```python
from build123d import *

# Parameters (mm, degrees)
OBJ1_R                     = 2.75
OBJ1_DEPTH                 = 8
OBJ2                     = 2.75
OBJ3                 = 8
OBJ4_PLACEMENT_ANGLE        = 90
TBOLT_SHAFT_R                    = 2
TBOLT_SHAFT_DEPTH                = 20
TBOLT_SHAFT_ROLL_ANGLE           = 90
UP_SEP_W                         = 16
UP_SEP_H                         = 1.2
UP_SEP_DEPTH                     = 13.8
SHAFT_HOLE_R                     = 4
SHAFT_HOLE_DEPTH                 = 16
SHAFT_HOLE_PITCH_ANGLE           = 90
TBOLT_HEAD_R                     = 3.85
TBOLT_HEAD_DEPTH                 = 5.4
TBOLT_HEAD_ROLL_ANGLE            = 90
SIDE_BOX_L_W                     = 14
SIDE_BOX_L_H                     = 12
SIDE_BOX_L_DEPTH                 = 26.8
SIDE_BOX_R_W                     = 14
SIDE_BOX_R_H                     = 12
SIDE_BOX_R_DEPTH                 = 26.8
TOTAL_BOX_W                      = 14
TOTAL_BOX_H                      = 42
TOTAL_BOX_DEPTH                  = 32.8
SK_SHAPE_W_HOLES_PLACEMENT_ANGLE = 90


with BuildPart() as obj1:
    # obj1 → obj1 (new body)
    with BuildSketch(Plane(origin=(7, -16, -1), x_dir=(1, 0, 0), z_dir=(0, 0, 1))):
        Circle(OBJ1_R)
    extrude(amount=OBJ1_DEPTH)


with BuildPart() as obj4:
    with BuildSketch(Plane(origin=(7, 16, -1), x_dir=(1, 0, 0), z_dir=(0, 0, 1))):
        Circle(OBJ2)
    extrude(amount=OBJ3)

    # obj4: union obj1
    add(obj1.part)


with BuildPart() as obj4_1:
    # obj4 placement: moved
    add(obj4.part.moved(Location((0, -7, 0))).rotate(Axis((0, -7, 0), (0, 0, 1)), OBJ4_PLACEMENT_ANGLE))


with BuildPart() as tbolt_shaft:
    # tbolt_shaft → tbolt_shaft (new body)
    with BuildSketch(Plane.XY):
        Circle(TBOLT_SHAFT_R)
    extrude(amount=TBOLT_SHAFT_DEPTH)


with BuildPart() as tbolt_shaft_1:
    # tbolt_shaft roll: moved
    add(tbolt_shaft.part.rotate(Axis((0, 0, 0), (1, 0, 0)), TBOLT_SHAFT_ROLL_ANGLE))


with BuildPart() as tbolt_shaft_2:
    # tbolt_shaft placement: moved
    add(tbolt_shaft_1.part.moved(Location((7, 10, 27.5))))


with BuildPart() as up_sep:
    # up_sep → up_sep (new body)
    with BuildSketch(Plane(origin=(-1, -0.6, 21), x_dir=(1, 0, 0), z_dir=(0, 0, 1))):
        with Locations((8, 0.6)):
            Rectangle(UP_SEP_W, UP_SEP_H)
    extrude(amount=UP_SEP_DEPTH)


with BuildPart() as shaft_hole:
    # shaft_hole → shaft_hole (new body)
    with BuildSketch(Plane.XY):
        Circle(SHAFT_HOLE_R)
    extrude(amount=SHAFT_HOLE_DEPTH)


with BuildPart() as shaft_hole_1:
    # shaft_hole pitch: moved
    add(shaft_hole.part.rotate(Axis((0, 0, 0), (0, 1, 0)), SHAFT_HOLE_PITCH_ANGLE))


with BuildPart() as shaft_hole_2:
    # shaft_hole placement: moved
    add(shaft_hole_1.part.moved(Location((-1, 0, 20))))


with BuildPart() as fuse_shaft_holes:
    # tbolt_head → tbolt_head (new body)
    with BuildSketch(Plane.XY):
        Circle(TBOLT_HEAD_R)
    extrude(amount=TBOLT_HEAD_DEPTH)


with BuildPart() as fuse_shaft_holes_1:
    # tbolt_head roll: moved
    add(fuse_shaft_holes.part.rotate(Axis((0, 0, 0), (1, 0, 0)), TBOLT_HEAD_ROLL_ANGLE))


with BuildPart() as fuse_shaft_holes_2:
    # tbolt_head placement: moved
    add(fuse_shaft_holes_1.part.moved(Location((7, 10, 27.5))))

    # fuse_shaft_holes: union tbolt_shaft, up_sep, shaft_hole
    add(tbolt_shaft_2.part)
    add(up_sep.part)
    add(shaft_hole_2.part)


with BuildPart() as side_box_l:
    # side_box_l → side_box_l (new body)
    with BuildSketch(Plane(origin=(0, -21, 6), x_dir=(1, 0, 0), z_dir=(0, 0, 1))):
        with Locations((7, 6)):
            Rectangle(SIDE_BOX_L_W, SIDE_BOX_L_H)
    extrude(amount=SIDE_BOX_L_DEPTH)


with BuildPart() as side_boxes:
    # side_box_r → side_box_r (new body)
    with BuildSketch(Plane(origin=(0, 9, 6), x_dir=(1, 0, 0), z_dir=(0, 0, 1))):
        with Locations((7, 6)):
            Rectangle(SIDE_BOX_R_W, SIDE_BOX_R_H)
    extrude(amount=SIDE_BOX_R_DEPTH)

    # side_boxes: union side_box_l
    add(side_box_l.part)


with BuildPart() as sky_x_y0:
    # total_box → total_box (new body)
    with BuildSketch(Plane(origin=(0, -21, 0), x_dir=(1, 0, 0), z_dir=(0, 0, 1))):
        with Locations((7, 21)):
            Rectangle(TOTAL_BOX_W, TOTAL_BOX_H)
    extrude(amount=TOTAL_BOX_DEPTH)

    # sk_shape: cut side_boxes
    add(side_boxes.part, mode=Mode.SUBTRACT)

    # sk_shape_w_holes: cut fuse_shaft_holes
    add(fuse_shaft_holes_2.part, mode=Mode.SUBTRACT)


with BuildPart() as sky_x_y0_1:
    # sk_shape_w_holes placement: moved
    add(sky_x_y0.part.moved(Location((0, -7, 0))).rotate(Axis((0, -7, 0), (0, 0, 1)), SK_SHAPE_W_HOLES_PLACEMENT_ANGLE))

    # sky_x_y0: cut obj4
    add(obj4_1.part, mode=Mode.SUBTRACT)


with BuildPart() as sky_x_y0_2:
    # sky_x_y0 placement: moved
    add(sky_x_y0_1.part.moved(Location((85.25, -56.5, -20))))


solid = sky_x_y0_2.part
```
Build history of the part. All positions in model axes, mm. A direction names the side the tool comes from. Coordinates: 2 decimals unless noted, no trailing zeros. Order: outer loops, then holes, each group sorted by start corner. A loop starts at its lowest first (then second) coordinate and runs counter-clockwise, first axis right, second up. Notation, with made-up numbers: M -32.5,-37.5 L 11.5,-37.5 A21 ccw 11.5,-22.5 Z; hole C 83.25,38.25 d9. An arc over 180 degrees is marked long. One line per question, with ' | ' between items. Start each with the question number.
1. Tool access for faces 1 (the face through (98.8, -58.2, -14)), 2 (the face through (85.85, -58.2, 9.3)), 3 (the face through (78.42, -52.83, 8.66)), 4 (the face through (73, -57, -14)), 5 (the face through (64.25, -57, -17)): list every direction of +Z, -Z, +X, -X, +Y, -Y with a clear straight run to the whole face (end or side of a thin tool).
2. Flat gauge pins, fed straight in: P1, Ø5, axis at y = -61.5, z = -5.5, coming from the -X side; P2, Ø7, axis at y = -60, z = 6.5, coming from the +X side; P3, Ø3.5, axis at y = -56.5, z = 7.5, coming from the +X side; P4, Ø4.5, axis at y = -55.5, z = 8.5, coming from the -X side. Where does each tip first touch, or does it go through?
3. Cut at D-D (z = -2). Write the cut outline in (x, y).
4. Cut at C-C (y = -56.5). Count the separate pieces of the cut face and the enclosed holes in it, plus the area to 3 significant figures.
5. Cut at B-B (x = 88). Write the cut outline in (y, z), plus the area to 3 significant figures.
6. Cut at A-A (z = 7.5). Write the cut outline in (x, y), plus the area to 3 significant figures.
7. Mould opens along Y. For faces 6 (the face through (86, -49.5, -11)), 7 (the face through (80.65, -54.8, 5.8)), 8 (the face through (86, -63.5, -11)), 9 (the face through (80, -57, 12.8)) say: +Y half, -Y half, draft (parallel to the pull), parting line (faces both ways), or undercut.
8. Wall check: line 1 along X through (y, z) = (-56.5, -17.7); line 2 along Y through (x, z) = (83.8, 7.5); line 3 along Z through (x, y) = (78.55, -56.5). Give the ranges that are in metal, low to high. Write a range as [from, to].
The answers:
1) face 1: +Z, +X, +Y, -Y | face 2: +Z, +Y, -Y | face 3: -X | face 4: +Z, -X, +Y, -Y | face 5: +Z, -Z, -X, +Y, -Y
2) P1: stops at x = 76.25 | P2: stops at x = 94.25 | P3: passes through | P4: stops at x = 80.65
3) outline: M 76.25,-63.5 L 81.79,-63.5 L 81.79,-49.5 L 76.25,-49.5 Z; M 88.71,-63.5 L 94.25,-63.5 L 94.25,-49.5 L 88.71,-49.5 Z
4) separate pieces: 5 | enclosed holes: 0 | area: 524 mm2
5) outline: M -63.5,-20 L -49.5,-20 L -49.5,-2.9 L -63.5,-2.9 Z; M -63.5,2.9 L -49.5,2.9 L -49.5,12.8 L -63.5,12.8 Z; hole C -56.5,7.5 d4 | area: 365 mm2
6) outline: M 76.25,-63.5 L 84.65,-63.5 L 84.65,-58.5 L 80.65,-58.5 L 80.65,-60.35 L 76.25,-60.35 Z; M 76.25,-52.65 L 80.65,-52.65 L 80.65,-54.5 L 84.65,-54.5 L 84.65,-49.5 L 76.25,-49.5 Z; M 85.85,-63.5 L 94.25,-63.5 L 94.25,-58.5 L 85.85,-58.5 Z; M 85.85,-54.5 L 94.25,-54.5 L 94.25,-49.5 L 85.85,-49.5 Z | area: 152 mm2
7) face 6: +Y half | face 7: undercut | face 8: -Y half | face 9: draft
8) line 1: x = [64.25, 66.5], [72, 98.5], [104, 106.25] | line 2: y = [-63.5, -58.5], [-54.5, -49.5] | line 3: z = [-20, 3.65], [11.35, 12.8]
